from build123d import *

# Parameters (mm, degrees)
F0_W     = 241.3
F0_H     = 152.4
F0_W_2   = 37.9902869463
F0_H_2   = 5.6053395383
F0_W_3   = 36.6508215666
F0_H_3   = 7.95059558
F0_W_4   = 211.6373926401
F0_H_4   = 6.9365315139
F0_H_5   = 7.6421592385
F0_R     = 25.4
F0_W_5   = 42.5071567297
F0_H_6   = 9.0162698179
F0_W_6   = 191.1512501538
F0_H_7   = 9.7504556179
F0_W_7   = 210.2212160826
F0_H_8   = 8.2425475121
F0_W_8   = 40.1230640709
F0_H_9   = 7.6498966664
F0_W_9   = 205.9216275811
F0_H_10  = 7.4272975326
F1_DEPTH = 2.54
F2_DEPTH = 2.54


with BuildPart() as f1:
    # F0 (on Front) → F1 (new body)
    with BuildSketch(Plane.XZ):
        with Locations((-32.7406, 25.5445336595)):
            Rectangle(F0_W, F0_H)
        with Locations((-118.0223450065, -2.8026697692)):
            Rectangle(F0_W_2, F0_H_2, mode=Mode.SUBTRACT)
        with Locations((-119.3700358272, 21.258618217)):
            Rectangle(F0_W_3, F0_H_3, mode=Mode.SUBTRACT)
        with BuildLine():
            ThreePointArc((-86.0117226839, 29.7584036313), (-58.2944755627, 35.3999965456), (-42.545, 11.9047336595))
            ThreePointArc((-42.545, 11.9047336595), (-77.5955244373, -11.5905292266), (-86.0117226839, 29.7584036313))
        make_face(mode=Mode.SUBTRACT)
        with Locations((-30.2752777934, -37.1060613543)):
            Rectangle(F0_W_4, F0_H_4, mode=Mode.SUBTRACT)
        with Locations((-30.2752777934, -20.3857226297)):
            Rectangle(F0_W_4, F0_H_5, mode=Mode.SUBTRACT)
        with Locations((0, 11.9047336595)):
            Circle(F0_R, mode=Mode.SUBTRACT)
        with Locations((54.2898401618, 4.508134909)):
            Rectangle(F0_W_5, F0_H_6, mode=Mode.SUBTRACT)
        with Locations((-33.6216446012, 91.3200601935)):
            Rectangle(F0_W_6, F0_H_7, mode=Mode.SUBTRACT)
        with Locations((-32.5848385692, 53.0171841383)):
            Rectangle(F0_W_7, F0_H_8, mode=Mode.SUBTRACT)
        with Locations((55.4818864912, 30.6309619918)):
            Rectangle(F0_W_8, F0_H_9, mode=Mode.SUBTRACT)
        with Locations((-30.7491086423, 75.0639848411)):
            Rectangle(F0_W_9, F0_H_10, mode=Mode.SUBTRACT)
    extrude(amount=F1_DEPTH)

    # F0 (on Front) → F2 (join)
    with BuildSketch(Plane.XZ):
        with Locations((-32.7406, 25.5445336595)):
            Rectangle(F0_W, F0_H)
        with Locations((-118.0223450065, -2.8026697692)):
            Rectangle(F0_W_2, F0_H_2, mode=Mode.SUBTRACT)
        with Locations((-119.3700358272, 21.258618217)):
            Rectangle(F0_W_3, F0_H_3, mode=Mode.SUBTRACT)
        with BuildLine():
            ThreePointArc((-86.0117226839, 29.7584036313), (-58.2944755627, 35.3999965456), (-42.545, 11.9047336595))
            ThreePointArc((-42.545, 11.9047336595), (-77.5955244373, -11.5905292266), (-86.0117226839, 29.7584036313))
        make_face(mode=Mode.SUBTRACT)
        with Locations((-30.2752777934, -37.1060613543)):
            Rectangle(F0_W_4, F0_H_4, mode=Mode.SUBTRACT)
        with Locations((-30.2752777934, -20.3857226297)):
            Rectangle(F0_W_4, F0_H_5, mode=Mode.SUBTRACT)
        with Locations((0, 11.9047336595)):
            Circle(F0_R, mode=Mode.SUBTRACT)
        with Locations((54.2898401618, 4.508134909)):
            Rectangle(F0_W_5, F0_H_6, mode=Mode.SUBTRACT)
        with Locations((-33.6216446012, 91.3200601935)):
            Rectangle(F0_W_6, F0_H_7, mode=Mode.SUBTRACT)
        with Locations((-32.5848385692, 53.0171841383)):
            Rectangle(F0_W_7, F0_H_8, mode=Mode.SUBTRACT)
        with Locations((55.4818864912, 30.6309619918)):
            Rectangle(F0_W_8, F0_H_9, mode=Mode.SUBTRACT)
        with Locations((-30.7491086423, 75.0639848411)):
            Rectangle(F0_W_9, F0_H_10, mode=Mode.SUBTRACT)
    extrude(amount=F2_DEPTH)


solid = f1.part
Design review of the part built by this model. Coordinates are the model's own, in mm. Give positions to 0.01 mm unless a question says otherwise; leave off trailing zeros. Order: outer loops, then holes, each group sorted by start corner. A loop starts at its lowest first (then second) coordinate and runs counter-clockwise, first axis right, second up.
1. Add section D-D, the plane x = 47.5. State how many separate pieces and enclosed holes the cut face has, then the cut area to 3 significant figures.
Solution:
separate pieces: 8
enclosed holes: 0
area: 243 mm2
2. Add section B-B, the plane x = -36. State the section outline as (y, z) points.
Solution:
outline: (-2.54, -50.66) - (0, -50.66) - (0, -40.57) - (-2.54, -40.57) - close; (-2.54, -33.64) - (0, -33.64) - (0, -24.21) - (-2.54, -24.21) - close; (-2.54, -16.56) - (0, -16.56) - (0, 48.9) - (-2.54, 48.9) - close; (-2.54, 57.14) - (0, 57.14) - (0, 71.35) - (-2.54, 71.35) - close; (-2.54, 78.78) - (0, 78.78) - (0, 86.44) - (-2.54, 86.44) - close; (-2.54, 96.2) - (0, 96.2) - (0, 101.74) - (-2.54, 101.74) - close
3. Add section C-C, the plane x = 0. State the section outline as (y, z) points.
Solution:
outline: (-2.54, -50.66) - (0, -50.66) - (0, -40.57) - (-2.54, -40.57) - close; (-2.54, -33.64) - (0, -33.64) - (0, -24.21) - (-2.54, -24.21) - close; (-2.54, -16.56) - (0, -16.56) - (0, -13.5) - (-2.54, -13.5) - close; (-2.54, 37.3) - (0, 37.3) - (0, 48.9) - (-2.54, 48.9) - close; (-2.54, 57.14) - (0, 57.14) - (0, 71.35) - (-2.54, 71.35) - close; (-2.54, 78.78) - (0, 78.78) - (0, 86.44) - (-2.54, 86.44) - close; (-2.54, 96.2) - (0, 96.2) - (0, 101.74) - (-2.54, 101.74) - close
4. Mouldability with a two-part tool opening along Z and no side actions: class faces 1 (the flat face through (-34, 0, 27)), 2 (the cylindrical face through (-20.157, -1.252, -3.551)) as +Z half, -Z half, draft (parallel to the pull), parting line (faces both ways), or undercut.
Solution:
face 1: draft
face 2: undercut
5. Add section A-A, the plane z = 75. State the section outline as (x, y) points, then the cut area to 3 significant figures.
Solution:
outline: (-153.39, -2.54) - (-133.71, -2.54) - (-133.71, 0) - (-153.39, 0) - close; (72.21, -2.54) - (87.91, -2.54) - (87.91, 0) - (72.21, 0) - close
area: 89.9 mm2
6. To check wall thickness, follow L1, parallel to X at y = -1.3, z = -36.5; L2, parallel to X at y = -2.1, z = 56; L3, parallel to X at y = -1.05, z = 28. State the ranges of each line that lie inside material, in increasing order.
Solution:
L1: x = -153.39 to -136.09, 75.54 to 87.91
L2: x = -153.39 to -137.7, 72.53 to 87.91
L3: x = -153.39 to -87.59, -48.3 to -19.65, 19.65 to 35.42, 75.54 to 87.91
